Input: part model. Units: mm. Frame: model coordinates. Coordinates: 2 decimals unless noted, no trailing zeros. Order: outer loops, then holes, each group sorted by start corner. A loop starts at its lowest first (then second) coordinate and runs counter-clockwise, first axis right, second up. Notation, with made-up numbers: M 8,41 L 53,41 A33 ccw 53,75 Z; hole C 33.25,60.5 d11. An arc over 180 degrees is marked long. One line per item, written item: value.
```python
from build123d import *

# Parameters (mm, degrees)
ESBO_O1_R                                   = 3
RESSALTO_EXTRUS_O1_DEPTH                    = 45
BROCA_DE_ROSQUEAR_PARA_TARRAXA_DE_M31_D     = 2.5
BROCA_DE_ROSQUEAR_PARA_TARRAXA_DE_M31_DEPTH = 8
BROCA_DE_ROSQUEAR_PARA_TARRAXA_DE_M31_TIP   = 0.751075774
BROCA_DE_ROSQUEAR_PARA_TARRAXA_DE_M32_D     = 2.5
BROCA_DE_ROSQUEAR_PARA_TARRAXA_DE_M32_DEPTH = 8
BROCA_DE_ROSQUEAR_PARA_TARRAXA_DE_M32_TIP   = 0.751075774


with BuildPart() as part:
    # Esboço1 → Ressalto-extrusão1 (new body)
    with BuildSketch(Plane.XY):
        with Locations(Location((0, 0, 0), (0, 0, 180))):
            Circle(ESBO_O1_R)
    extrude(amount=RESSALTO_EXTRUS_O1_DEPTH)

    # Broca de rosquear para tarraxa de M31
    with Locations(Plane.XY.offset(45)):
        with Locations((0, 0)):
            Hole(BROCA_DE_ROSQUEAR_PARA_TARRAXA_DE_M31_D / 2, depth=BROCA_DE_ROSQUEAR_PARA_TARRAXA_DE_M31_DEPTH)
            with Locations((0, 0, -(BROCA_DE_ROSQUEAR_PARA_TARRAXA_DE_M31_DEPTH + BROCA_DE_ROSQUEAR_PARA_TARRAXA_DE_M31_TIP / 2))):  # 118° drill point
                Cone(0, BROCA_DE_ROSQUEAR_PARA_TARRAXA_DE_M31_D / 2, BROCA_DE_ROSQUEAR_PARA_TARRAXA_DE_M31_TIP, mode=Mode.SUBTRACT)

    # Broca de rosquear para tarraxa de M32
    with Locations(Plane(origin=(0, 0, 0), x_dir=(-1, 0, 0), z_dir=(0, 0, -1))):
        with Locations((0, 0)):
            Hole(BROCA_DE_ROSQUEAR_PARA_TARRAXA_DE_M32_D / 2, depth=BROCA_DE_ROSQUEAR_PARA_TARRAXA_DE_M32_DEPTH)
            with Locations((0, 0, -(BROCA_DE_ROSQUEAR_PARA_TARRAXA_DE_M32_DEPTH + BROCA_DE_ROSQUEAR_PARA_TARRAXA_DE_M32_TIP / 2))):  # 118° drill point
                Cone(0, BROCA_DE_ROSQUEAR_PARA_TARRAXA_DE_M32_D / 2, BROCA_DE_ROSQUEAR_PARA_TARRAXA_DE_M32_TIP, mode=Mode.SUBTRACT)


solid = part.part
```
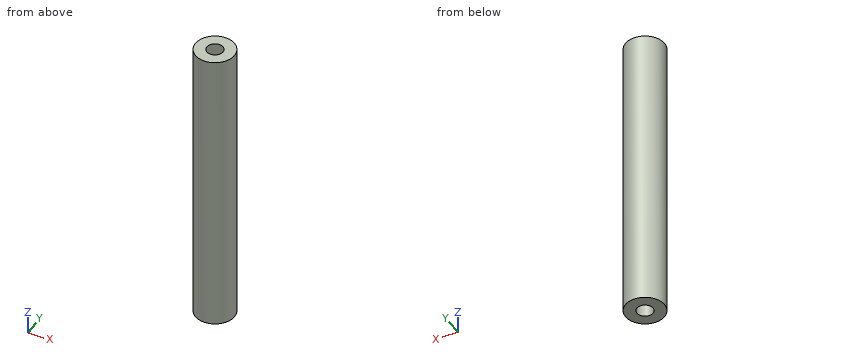
(1) Cut plane D-D on x = -2.3. Output: boundary loops of the cut face in (y, z).
Data:
outline: M -1.93,0 L 1.93,0 L 1.93,45 L -1.93,45 Z
(2) First-contact query: pin 1 (2 mm diameter, centred on x = 0, y = 0, fed in from -Z); pin 2 (1 mm diameter, centred on x = -1.5, z = 6, fed in from +Y); pin 3 (1.5 mm diameter, centred on x = -2, z = 5.5, fed in from -Y). Flat tips, straight axial feed; report the tip coordinate or a pass-through.
Data:
pin 1: stops at z = 8.15
pin 2: stops at y = 2.83
pin 3: stops at y = -2.73
(3) Ray query, line 1 (Y direction, x = 0, z = 2.5); line 2 (X direction, y = -0.15, z = 15). Return the intervals inside material, ascending. Write a range as from..to.
Data:
line 1: y = -3..-1.25, 1.25..3
line 2: x = -3..3
(4) Cut plane C-C on z = 12. Output: boundary loops of the cut face in (x, y).
Data:
outline: C 0,0 d6
(5) Cut plane A-A on z = 39. Output: boundary loops of the cut face in (x, y), plus the area to 3 significant figures.
Data:
outline: C 0,0 d6; hole C 0,0 d2.5
area: 23.4 mm2
(6) Cut plane B-B on y = 1.8. Output: boundary loops of the cut face in (x, z), plus the area to 3 significant figures.
Data:
outline: M -2.4,0 L 2.4,0 L 2.4,45 L -2.4,45 Z
area: 216 mm2
